The model under review builds one solid part; all positions refer to its coordinate system, in mm. A direction names the side the tool comes from. Coordinates: 2 decimals unless noted, no trailing zeros. Loops run counter-clockwise (first coordinate to the right, second up) from the corner with the lowest first, then second, coordinate; pieces in that order, holes last. Notation, with made-up numbers: M 12,60 L 23,60 A14 ccw 23,79 Z; hole C 61,76.25 d5. An arc over 180 degrees is marked long. Return JSON: item names as keys, results as strings.
```python
from build123d import *

# Parameters (mm, degrees)
SKETCH1_W           = 4
SKETCH1_H           = 4
BOSS_EXTRUDE1_DEPTH = 100
SKETCH2_W           = 4
SKETCH2_H           = 5
BOSS_EXTRUDE2_DEPTH = 25
FILLET1_R           = 10
FILLET3_R           = 4
FILLET4_R           = 2


with BuildPart() as part:
    # Sketch1 → Boss-Extrude1 (new body)
    with BuildSketch(Plane(origin=(0, 0, 0), x_dir=(1, 0, 0), z_dir=(0, 1, 0))):
        with Locations((2, 2)):
            Rectangle(SKETCH1_W, SKETCH1_H)
    extrude(amount=BOSS_EXTRUDE1_DEPTH)

    # Sketch2 → Boss-Extrude2 (add)
    with BuildSketch(Plane(origin=(4, 0, 0), x_dir=(0, 0, -1), z_dir=(1, 0, 0))):
        with Locations((2, 97.5)):
            Rectangle(SKETCH2_W, SKETCH2_H)
    extrude(amount=BOSS_EXTRUDE2_DEPTH)

    # Fillet1
    fillet1_edges = [part.edges().sort_by_distance(p)[0] for p in [
        (4, 95, -2),
    ]]
    fillet(fillet1_edges, radius=FILLET1_R)

    # Fillet3
    # the kernel refuses this fillet: 4 mm, written as the material it takes off along each edge
    with BuildSketch(Plane(origin=(39, 100, -4), x_dir=(0, 0, 1), z_dir=(-1, 0, 0)), Plane(origin=(39, 100, 0), x_dir=(0, -1, 0), z_dir=(-1, 0, 0))) as fillet3_piece_1:
        with BuildLine():
            CenterArc((FILLET3_R, -FILLET3_R), FILLET3_R, 90, 90)
            Line((0, -FILLET3_R), (0, 0))
            Line((0, 0), (FILLET3_R, 0))
        make_face()
    extrude(amount=49, mode=Mode.SUBTRACT)
    with BuildSketch(Plane(origin=(29, 100, -14), x_dir=(0, -1, 0), z_dir=(0, 0, 1)), Plane(origin=(0, 100, -14), x_dir=(1, 0, 0), z_dir=(0, 0, 1))) as fillet3_piece_2:
        with BuildLine():
            CenterArc((FILLET3_R, -FILLET3_R), FILLET3_R, 90, 90)
            Line((0, -FILLET3_R), (0, 0))
            Line((0, 0), (FILLET3_R, 0))
        make_face()
    extrude(amount=24, mode=Mode.SUBTRACT)

    # Fillet4
    # the kernel refuses this fillet: 2 mm, written as the material it takes off along each edge
    with BuildSketch(Plane(origin=(29, 95, 7.618721628), x_dir=(-1, 0, 0), z_dir=(0, 0, -1))) as fillet4_piece_1:
        with BuildLine():
            CenterArc((2.267949192, 2), FILLET4_R, 150, 120)
            Line((0.535898385, 3), (0.362693304, 3.1))
            ThreePointArc((0.362693304, 3.1), (-0.2, 1), (-0.2, 0))
            Line((-0.2, 0), (0, -0.2))
            Line((0, -0.2), (2.267949192, -0.2))
            Line((2.267949192, -0.2), (2.267949192, 0))
        make_face()
    extrude(amount=19.237443256, mode=Mode.SUBTRACT)


solid = part.part
```
1. Add section B-B on y = 79.5. Give the boundary of the cut face in (x, z), plus the area to 3 significant figures.
Check values:
{"outline": "M 0,-4 L 4,-4 L 4,0 L 0,0 Z", "area": "16.0 mm²"}
2. Add section C-C on x = 11.75. Give the boundary of the cut face in (y, z), plus the area to 3 significant figures.
Check values:
{"outline": "M 94.74,-4 L 96,-4 A4 ccw 99.46,-2 A4 ccw 96,0 L 94.74,0 Z", "area": "14.9 mm²"}
3. Add section D-D on y = 90. Give the boundary of the cut face in (x, z), plus the area to 3 significant figures.
Check values:
{"outline": "M 0,-4 L 5.34,-4 L 5.34,0 L 0,0 Z", "area": "21.4 mm²"}
4. Insertion check: pin 1 Ø2 at (x, y) = (4.5, 21.5) entering from -Z; pin 2 Ø2 at (y, z) = (52, -1.5) entering from +X; pin 3 Ø2 at (x, z) = (19.5, -1.5) entering from -Y; pin 4 Ø8 at (x, y) = (17.5, 89) entering from +Z. Each pin has a flat end and moves straight along its axis. Give the tip position at first contact, or say it passes through.
Check values:
{"pin 1": "z = -4", "pin 2": "x = 4", "pin 3": "y = 95", "pin 4": "through"}
5. Add section A-A on x = 17. Give the boundary of the cut face in (y, z).
Check values:
{"outline": "M 95,-4 L 96,-4 A4 ccw 99.46,-2 A4 ccw 96,0 L 95,0 Z"}
6. Machinability: for faces 1 (the face through (20, 95, -2)), 2 (the face through (0, 47, -2)), which of the approach directions +Z, -Z, +X, -X, +Y, -Y give a long, thin tool a straight path to every point of the face, cutting with its end or side? Answer none if there is none.
Check values:
{"face 1": "+Z, -Z, +X, -Y", "face 2": "+Z, -Z, -X, +Y, -Y"}
7. To check wall thickness, follow line 1 (X direction, y = 7.5, z = -2.4); line 2 (Y direction, x = 27.75, z = -1.95); line 3 (X direction, y = 88, z = -3.4). State the ranges of each line that lie inside material, in increasing order.
Check values:
{"line 1": "0 to 4", "line 2": "95.28 to 98.9", "line 3": "0 to 4.46"}
